```python
from build123d import *

# Parameters (mm, degrees)
CUT_EXTRUDE1_START = 66
SKETCH2_R          = 14.5
CUT_EXTRUDE1_DEPTH = 66
SKETCH3_W          = 35
SKETCH3_H          = 2
CUT_EXTRUDE2_DEPTH = 3


with BuildPart() as part:
    # Sketch1 → Revolve1 (revolve)
    with BuildSketch(Plane(origin=(0, 0, 0), x_dir=(0, 0, -1), z_dir=(1, 0, 0))):
        Polygon((-16, 3.37389395), (-40, 3.37389395), (-40, -0.62610605), (-14.5, -0.62610605), (-14, -0.62610605), (-14, -36.62610605), (-13, -36.62610605), (-13, -0.62610605), (-13, 11.37389395), (-14.5, 11.37389395), (-14.5, 23.37389395), (-16, 23.37389395), align=None)
    revolve1 = revolve(axis=Axis((0, 28.058626224, 0), (0, -1, 0)))

    # Mirror3: Revolve1 across plane
    add(revolve1.mirror(Plane.ZX.offset(13.37389395)))

    # Sketch2 → Cut-Extrude1 (cut)
    with BuildSketch(Plane(origin=(0, 11.37389395, 0), x_dir=(1, 0, 0), z_dir=(0, 1, 0)).offset(CUT_EXTRUDE1_START)):
        with Locations(Location((0, 0, 0), (0, 0, 270))):
            Circle(SKETCH2_R)
    extrude(amount=-CUT_EXTRUDE1_DEPTH, mode=Mode.SUBTRACT)

    # Sketch3 → Cut-Extrude2 (cut)
    with BuildSketch(Plane(origin=(0, 27.37389395, 0), x_dir=(1, 0, 0), z_dir=(0, 1, 0))):
        Rectangle(SKETCH3_W, SKETCH3_H)
    extrude(amount=-CUT_EXTRUDE2_DEPTH, mode=Mode.SUBTRACT)


solid = part.part
```
Check sheet for the modelled part. Datum: model origin and axes. Units: mm. A direction names the side the tool comes from. Coordinates: 2 decimals unless noted, no trailing zeros. Write each loop counter-clockwise with the first axis right and the second up, starting at its lowest first coordinate (ties: lowest second). Pieces come first, ordered by that corner, then holes. Notation, with made-up numbers: (42.5, 51.25) -> (56.5, 51.25) arc R11 cw to (56.5, 55.25) -> close; hole circle Ø1 at (-36, -29). An arc over 180 degrees is marked (long way). Use a Markdown table: item, result.
1. Scan lines: line 1 along Y through (x, z) = (-9.5, -26.5); line 2 along Z through (x, y) = (0, -21); line 3 along Z through (x, y) = (0, 24). Record each from-to range of solid material in increasing order.
Reported:
| item | result |
|---|---|
| line 1 | y = -0.63 to 3.37, 23.37 to 27.37 |
| line 2 | z = -14 to -13, 13 to 14 |
| line 3 | z = -40 to -14.5, 14.5 to 40 |
2. Go/stop test with flat-tipped pins: pin 1 Ø1.5 at (x, y) = (16, 25.5) entering from +Z; pin 2 Ø14.5 at (x, z) = (-6, -5) entering from +Y; pin 3 Ø1 at (y, z) = (26.5, -0.5) entering from -X; pin 4 Ø2.5 at (x, y) = (16.5, 25.5) entering from -Z. Record where each tip stops, or that it passes through.
Reported:
| item | result |
|---|---|
| pin 1 | stops at z = 36.98 |
| pin 2 | stops at y = 27.37 |
| pin 3 | stops at x = -40 |
| pin 4 | stops at z = -36.98 |
3. Sectioned sample at A-A (x = 0). Enter the section's corners in (y, z), plus the area to 3 significant figures.
Reported:
| item | result |
|---|---|
| outline | (-36.63, -14) -> (-0.63, -14) -> (-0.63, -40) -> (3.37, -40) -> (3.37, -16) -> (23.37, -16) -> (23.37, -40) -> (27.37, -40) -> (27.37, -14.5) -> (11.37, -14.5) -> (11.37, -13) -> (-36.63, -13) -> close; (-36.63, 13) -> (11.37, 13) -> (11.37, 14.5) -> (27.37, 14.5) -> (27.37, 40) -> (23.37, 40) -> (23.37, 16) -> (3.37, 16) -> (3.37, 40) -> (-0.63, 40) -> (-0.63, 14) -> (-36.63, 14) -> close |
| area | 576 mm2 |
4. Release check for a two-part mould opening along Z. For faces 1 (the flat face through (-17.5, 26, 0)), 2 (the flat face through (-16, 26, 1)), 3 (the cylindrical face through (5.362, -18.878, 12.932)), 4 (the flat face through (-1, 27.374, 17)) record: pulls with the +Z half, pulls with the -Z half, needs draft (parallel to the pull), parting line crosses it, or undercut.
Reported:
| item | result |
|---|---|
| face 1 | undercut |
| face 2 | undercut |
| face 3 | parting line crosses it |
| face 4 | needs draft |
5. Tool access check on faces 5 (the cylindrical face through (7.91, -12.29, -10.316)), 6 (the flat face through (9.3, -36.626, 9.3)), 7 (the cylindrical face through (-5.554, 19.486, 13.394)), 8 (the flat face through (-1, -0.626, 17)), 9 (the flat face through (-1, 23.374, -17)). Record the directions out of +Z, -Z, +X, -X, +Y, -Y that give a thin tool (end or side, any length) a straight path to the whole face; none if there is none.
Reported:
| item | result |
|---|---|
| face 5 | +Y, -Y |
| face 6 | +Z, -Z, +X, -X, -Y |
| face 7 | +Y |
| face 8 | -Y |
| face 9 | none |
6. Sectioned sample at D-D (x = -33.5). Enter the section's corners in (y, z).
Reported:
| item | result |
|---|---|
| outline | (-0.63, -21.86) -> (3.37, -21.86) -> (3.37, 21.86) -> (-0.63, 21.86) -> close; (23.37, -21.86) -> (27.37, -21.86) -> (27.37, 21.86) -> (23.37, 21.86) -> close |
7. Sectioned sample at C-C (y = 10). Enter the section's corners in (x, z).
Reported:
| item | result |
|---|---|
| outline | circle Ø32 at (0, 0); hole circle Ø26 at (0, 0) |
8. Sectioned sample at B-B (z = -5). Enter the section's corners in (x, y), plus the area to 3 significant figures.
Reported:
| item | result |
|---|---|
| outline | (-39.69, -0.63) -> (-13.08, -0.63) -> (-13.08, -36.63) -> (-12, -36.63) -> (-12, 11.37) -> (-13.61, 11.37) -> (-13.61, 27.37) -> (-39.69, 27.37) -> (-39.69, 23.37) -> (-15.2, 23.37) -> (-15.2, 3.37) -> (-39.69, 3.37) -> close; (12, -36.63) -> (13.08, -36.63) -> (13.08, -0.63) -> (39.69, -0.63) -> (39.69, 3.37) -> (15.2, 3.37) -> (15.2, 23.37) -> (39.69, 23.37) -> (39.69, 27.37) -> (13.61, 27.37) -> (13.61, 11.37) -> (12, 11.37) -> close |
| area | 597 mm2 |
